from build123d import *

# Parameters (mm, degrees)
BASE_EXTRUSION_DEPTH = 2


with BuildPart() as part:
    # Esquisse1 → Base-Extrusion (new body)
    with BuildSketch(Plane.XY):
        with BuildLine():
            Line((-16.5, -22.5), (-10.5, -22.5))
            ThreePointArc((-10.5, -22.5), (-8.707157086, -23.094648823), (-7.625055458, -24.642857143))
            ThreePointArc((-7.625055458, -24.642857143), (-7.444705186, -24.900891863), (-7.145898034, -25))
            Line((-7.145898034, -25), (7.145898034, -25))
            ThreePointArc((7.145898034, -25), (7.444705186, -24.900891863), (7.625055458, -24.642857143))
            ThreePointArc((7.625055458, -24.642857143), (8.707157086, -23.094648823), (10.5, -22.5))
            Line((10.5, -22.5), (16.5, -22.5))
            ThreePointArc((16.5, -22.5), (17.560660172, -22.060660172), (18, -21))
            Line((18, -21), (18, 21))
            ThreePointArc((18, 21), (17.560660172, 22.060660172), (16.5, 22.5))
            Line((16.5, 22.5), (10.5, 22.5))
            ThreePointArc((10.5, 22.5), (8.707157086, 23.094648823), (7.625055458, 24.642857143))
            ThreePointArc((7.625055458, 24.642857143), (7.444705186, 24.900891863), (7.145898034, 25))
            Line((7.145898034, 25), (-7.145898034, 25))
            ThreePointArc((-7.145898034, 25), (-7.444705186, 24.900891863), (-7.625055458, 24.642857143))
            ThreePointArc((-7.625055458, 24.642857143), (-8.707157086, 23.094648823), (-10.5, 22.5))
            Line((-10.5, 22.5), (-16.5, 22.5))
            ThreePointArc((-16.5, 22.5), (-17.560660172, 22.060660172), (-18, 21))
            Line((-18, 21), (-18, -21))
            ThreePointArc((-18, -21), (-17.560660172, -22.060660172), (-16.5, -22.5))
        make_face()
        with BuildLine():
            Line((-16, -20.5), (-10.5, -20.5))
            ThreePointArc((-10.5, -20.5), (-8, -21.169872981), (-6.169872981, -23))
            Line((-6.169872981, -23), (-3, -23))
            Line((-3, -23), (-3, -23.903020069))
            Line((-3, -23.903020069), (3, -23.903020069))
            Line((3, -23.903020069), (3, -23))
            Line((3, -23), (6.169872981, -23))
            ThreePointArc((6.169872981, -23), (8, -21.169872981), (10.5, -20.5))
            Line((10.5, -20.5), (16, -20.5))
            Line((16, -20.5), (16, 20.5))
            Line((16, 20.5), (10.5, 20.5))
            ThreePointArc((10.5, 20.5), (8, 21.169872981), (6.169872981, 23))
            Line((6.169872981, 23), (3, 23))
            Line((3, 23), (3, 23.903020069))
            Line((3, 23.903020069), (-3, 23.903020069))
            Line((-3, 23.903020069), (-3, 23))
            Line((-3, 23), (-6.169872981, 23))
            ThreePointArc((-6.169872981, 23), (-8, 21.169872981), (-10.5, 20.5))
            Line((-10.5, 20.5), (-16, 20.5))
            Line((-16, 20.5), (-16, -20.5))
        make_face(mode=Mode.SUBTRACT)
    extrude(amount=BASE_EXTRUSION_DEPTH)


solid = part.part
Input: part model. Units: mm. Frame: model coordinates. A direction names the side the tool comes from. Coordinates: 2 decimals unless noted, no trailing zeros. Order: outer loops, then holes, each group sorted by start corner. A loop starts at its lowest first (then second) coordinate and runs counter-clockwise, first axis right, second up.
1. Cut plane B-B, the plane x = 1.5. Return loops of the section in (y, z).
Checked values:
outline: (-25, 0) - (-23.9, 0) - (-23.9, 2) - (-25, 2) - close; (23.9, 0) - (25, 0) - (25, 2) - (23.9, 2) - close
2. Access query for faces 1 (the cylindrical face through (-8.7, 23.1, 1)), 2 (the flat face through (-5, 23, 1)), 3 (the flat face through (14, 22.5, 1)). Directions: +Z, -Z, +X, -X, +Y, -Y. A direction counts if a zero-diameter tool reaches every point of the face in a straight line with its end or side. Return the directions, or none.
Checked values:
face 1: +Z, -Z, -X, +Y
face 2: +Z, -Z
face 3: +Z, -Z, +X, +Y
3. Draft query along Y for faces 4 (the cylindrical face through (-8.032, -21.152, 0.986)), 5 (the flat face through (-5, -23, 1)), 6 (the flat face through (13, -22.5, 1)), 7 (the flat face through (18, 0, 1)). Return one class per face: +Y half, -Y half, draft (parallel to the pull), parting line (faces both ways), or undercut.
Checked values:
face 4: undercut
face 5: undercut
face 6: -Y half
face 7: draft
4. Cut plane A-A, the plane y = 12.5. Return loops of the section in (x, z).
Checked values:
outline: (-18, 0) - (-16, 0) - (-16, 2) - (-18, 2) - close; (16, 0) - (18, 0) - (18, 2) - (16, 2) - close
5. Ray query, line 1 along Y through (x, z) = (12.5, 1.1); line 2 along Y through (x, z) = (2, 0.5); line 3 along X through (y, z) = (16.5, 0.45). Return the intervals inside material, ascending.
Checked values:
line 1: y = -22.5 to -20.5, 20.5 to 22.5
line 2: y = -25 to -23.9, 23.9 to 25
line 3: x = -18 to -16, 16 to 18
6. Contact query for flat-ended pins moving along their axis: P1, Ø0.6, axis at x = 13.5, z = 1, coming from the +Y side; P2, Ø1, axis at x = -12.5, z = 1.5, coming from the -Y side; P3, Ø1, axis at y = 23.5, z = 1.5, coming from the +X side. Output: stop coordinate, or through.
Checked values:
P1: stops at y = 22.5
P2: stops at y = -22.5
P3: stops at x = 8.84
